For this review, take the finished solid that the model builds, in its own axes (mm). A direction names the side the tool comes from. Give positions to 0.01 mm unless a question says otherwise; leave off trailing zeros. Loops run counter-clockwise (first coordinate to the right, second up) from the corner with the lowest first, then second, coordinate; pieces in that order, holes last. Notation, with made-up numbers: (-20.75, 4) - (29.25, 4) arc R26 ccw to (29.25, 18) - close; hole circle Ø11 at (-16, 38.5). An arc over 180 degrees is marked (long way). Answer in a Markdown table with one row per item.
```python
from build123d import *

# Parameters (mm, degrees)
CUT_EXTRUDE1_DEPTH = 1.84404
SKETCH5_R          = 2.291358881
CUT_EXTRUDE2_DEPTH = 1.84404
CUT_EXTRUDE2_DRAFT = -60
FILLET1_R          = 0.16764


with BuildPart() as part:
    # Sketch3 → Revolve1 (revolve)
    with BuildSketch(Plane(origin=(0, 0, 0), x_dir=(0, 0, -1), z_dir=(1, 0, 0))):
        with BuildLine():
            Line((-14.3764, 0), (-14.3764, 2.778125))
            ThreePointArc((-14.3764, 2.778125), (-13.182024687, 4.401074199), (-11.52652, 5.5499))
            Line((-11.52652, 5.5499), (-11.0236, 5.461221635))
            Line((-11.0236, 5.461221635), (-11.0236, 3.175))
            Line((-11.0236, 3.175), (13.4239, 3.175))
            Line((13.4239, 3.175), (14.3764, 2.2225))
            Line((14.3764, 2.2225), (14.3764, 0))
            Line((14.3764, 0), (-14.3764, 0))
        make_face()
    revolve(axis=Axis((0, 0, 14.3764), (0, 0, -1)))

    # Sketch4 → Cut-Extrude1 (cut)
    with BuildSketch(Plane.XY.offset(14.3764)):
        Polygon((-1.984375, -1.14567944), (0, -2.291358881), (1.984375, -1.14567944), (1.984375, 1.14567944), (0, 2.291358881), (-1.984375, 1.14567944), align=None)
    extrude(amount=-CUT_EXTRUDE1_DEPTH, mode=Mode.SUBTRACT)


with BuildPart() as cut_extrude2_tool:
    # Sketch5 → Cut-Extrude2 (with draft: the straight prism first)
    with BuildSketch(Plane.XY.offset(14.3764)):
        Circle(SKETCH5_R)
    extrude(amount=-CUT_EXTRUDE2_DEPTH)
    # Cut-Extrude2: the draft: its side faces are tilted about the plane it starts from
    cut_extrude2_sides = [cut_extrude2_tool.faces().sort_by_distance(p)[0] for p in [
        (-2.291358881, 0, 13.45438),
    ]]
    draft(cut_extrude2_sides, Plane.XY.offset(14.3764), CUT_EXTRUDE2_DRAFT)


with BuildPart() as part_1:
    add(part.part)

    # Cut-Extrude2: cut by cut_extrude2_tool
    add(cut_extrude2_tool.part, mode=Mode.SUBTRACT)

    # Fillet1
    fillet1_edges = [part_1.edges().sort_by_distance(p)[0] for p in [
        (0, -5.461221635, 11.0236),
        (0, -5.5499, 11.52652),
    ]]
    fillet(fillet1_edges, radius=FILLET1_R)


solid = part_1.part
```
1. Mouldability with a two-part tool opening along Y and no side actions: class faces 3 (the face through (1.06, -1.86, 14.29)), 4 (the face through (0, 0, -14.376)), 5 (the face through (-3.1, -0.69, -1.37)) as released by +Y, released by -Y, zero draft, split by the parting line, or undercut.
Values:
| item | result |
|---|---|
| face 3 | undercut |
| face 4 | zero draft |
| face 5 | split by the parting line |
2. We need section A-A, the plane z = -4. Give the boundary of the cut face in (x, y) (3 decimals).
Values:
| item | result |
|---|---|
| outline | circle Ø6.35 at (0, 0) |
3. Wall thickness on line 1 (Z direction, x = -1.25, y = 1.5); line 2 (Z direction, x = -3.5, y = 0.25); line 3 (Y direction, x = -0.5, z = -9): over which ranges is each line inside the solid? List them lowest first. Write a range as [from, to].
Values:
| item | result |
|---|---|
| line 1 | z = [-14.38, 12.53] |
| line 2 | z = [11.02, 13.94] |
| line 3 | y = [-3.14, 3.14] |
4. Clearance check with flat-ended pins moving along their axes: pin 1 (1.5 mm diameter, centred on x = 2.5, y = -4.5, fed in from +Z); pin 2 (6 mm diameter, centred on y = -3, z = -3, fed in from +X) (3 decimals); pin 3 (1.5 mm diameter, centred on x = 2.5, y = -2.5, fed in from -Z). State where each tip first meets the part, or that it passes through.
Values:
| item | result |
|---|---|
| pin 1 | stops at z = 13.19 |
| pin 2 | stops at x = 3.175 |
| pin 3 | stops at z = -13.81 |
5. For faces 1 (the face through (-3.5, -0.1, 11.024)), 2 (the face through (-0.978, 1.727, 13.467)), list the 3-axis set-ups (+Z, -Z, +X, -X, +Y, -Y) from which the entire face can be reached by the end or side of a thin tool; tool diameter is ignored.
Values:
| item | result |
|---|---|
| face 1 | -Z |
| face 2 | +Z |
